Geometry: final body of the model. Coordinates: model frame, mm. A direction names the side the tool comes from. Coordinates: 2 decimals unless noted, no trailing zeros. Loops run counter-clockwise (first coordinate to the right, second up) from the corner with the lowest first, then second, coordinate; pieces in that order, holes last. Notation, with made-up numbers: (48, 7) - (70, 7) arc R13 cw to (70, 17) - close; hole circle Ø7 at (64.25, 68.5). An arc over 180 degrees is marked (long way). Put each result on its own line as item: value. Start each with the question number.
1) Section D-D on z = 30. Output: boundary loops of the cut face in (x, y).
2) Draft query along Z for faces 1 (the flat face through (5, 0, 3)), 2 (the flat face through (5, 13, 41.48)), 3 (the flat face through (-30, 16, 18.62)), 4 (the flat face through (0.86, 9, 4)). Return one class per face: +Z half, -Z half, draft (parallel to the pull), parting line (faces both ways), or undercut.
3) Section C-C on y = 17.78. Output: boundary loops of the cut face in (x, z).
4) Section A-A on y = 4.25. Output: boundary loops of the cut face in (x, z), and give its area (3 significant figures).
5) Reachability of faces 5 (the flat face through (-30, 16, 12.27)), 6 (the flat face through (5, 13, -34.72)), 7 (the flat face through (11, 9, -25.195)) from +Z, -Z, +X, -X, +Y, -Y: full face, straight path, thin tool, end or side. Return the list, or none.
6) Material intervals for line 1 along X through (y, z) = (11.5, -16); line 2 along Z through (x, y) = (-14.5, 14.25); line 3 along X through (y, z) = (12.75, 35.5), sorted ascending. Write a range as from..to.
7) Contact query for flat-ended pins moving along their axis: pin 1 Ø14 at (y, z) = (10.5, 4) entering from -X; pin 2 Ø4.5 at (y, z) = (17.78, -11.86) entering from -X; pin 3 Ø1.5 at (y, z) = (12.5, 5) entering from -X. Output: stop coordinate, or through.
8) Section B-B on x = 48.5. Output: boundary loops of the cut face in (y, z).
```python
from build123d import *

# Parameters (mm, degrees)
SKETCH1_W           = 101.6
SKETCH1_H           = 76.2
BOSS_EXTRUDE1_DEPTH = 25.4
SKETCH2_W           = 77.204847721
SKETCH2_H           = 71.12
CUT_EXTRUDE1_DEPTH  = 22.86
SKETCH3_W           = 73.394847721
SKETCH3_H           = 63.5
BOSS_EXTRUDE3_DEPTH = 12.7
SKETCH4_W           = 38.1
SKETCH4_H           = 15.24
CUT_EXTRUDE2_DEPTH  = 6.35
SKETCH7_R           = 2.535464608
CUT_EXTRUDE3_DEPTH  = 22.86
SKETCH8_W           = 6.35
SKETCH8_H           = 6.35
CUT_EXTRUDE5_DEPTH  = 17.78
SKETCH9_W           = 20.32
SKETCH9_H           = 57.15
CUT_EXTRUDE6_DEPTH  = 12.7
LPATTERN1_COUNT     = 3
LPATTERN1_PITCH     = 22.86


with BuildPart() as part:
    # Sketch1 → Boss-Extrude1 (new body)
    with BuildSketch(Plane(origin=(0, 0, 0), x_dir=(1, 0, 0), z_dir=(0, 1, 0))):
        with Locations((5.940322581, -3.37983871)):
            Rectangle(SKETCH1_W, SKETCH1_H)
    extrude(amount=BOSS_EXTRUDE1_DEPTH)

    # Sketch2 → Cut-Extrude1 (cut)
    with BuildSketch(Plane(origin=(0, 25.4, 0), x_dir=(1, 0, 0), z_dir=(0, 1, 0))):
        with Locations((15.59789872, -3.37983871)):
            Rectangle(SKETCH2_W, SKETCH2_H)
    extrude(amount=-CUT_EXTRUDE1_DEPTH, mode=Mode.SUBTRACT)

    # Sketch3 → Boss-Extrude3 (add)
    with BuildSketch(Plane(origin=(0, 2.54, 0), x_dir=(1, 0, 0), z_dir=(0, 1, 0))):
        with Locations((13.692898721, -3.37983871)):
            Rectangle(SKETCH3_W, SKETCH3_H)
    extrude(amount=BOSS_EXTRUDE3_DEPTH)

    # Sketch4 → Cut-Extrude2 (cut)
    with BuildSketch(Plane.ZY.offset(44.859677419)):
        with Locations((3.37983871, 13.97)):
            Rectangle(SKETCH4_W, SKETCH4_H)
    extrude(amount=-CUT_EXTRUDE2_DEPTH, mode=Mode.SUBTRACT)

    # Sketch7 → Cut-Extrude3 (cut)
    with BuildSketch(Plane.ZY.offset(44.859677419)):
        with Locations((-11.86016129, 17.78)):
            Circle(SKETCH7_R)
    extrude(amount=-CUT_EXTRUDE3_DEPTH, mode=Mode.SUBTRACT)

    # Sketch8 → Cut-Extrude5 (cut)
    with BuildSketch(Plane.ZY.offset(38.509677419)):
        with Locations((15.44483871, 15.875)):
            Rectangle(SKETCH8_W, SKETCH8_H)
    extrude(amount=-CUT_EXTRUDE5_DEPTH, mode=Mode.SUBTRACT)

    # Sketch9 → Cut-Extrude6 (cut)
    with BuildSketch(Plane(origin=(0, 15.24, 0), x_dir=(1, 0, 0), z_dir=(0, 1, 0))):
        with Locations((33.880322581, -3.37983871)):
            Rectangle(SKETCH9_W, SKETCH9_H)
    cut_extrude6 = extrude(amount=-CUT_EXTRUDE6_DEPTH, mode=Mode.SUBTRACT)

    # LPattern1: Cut-Extrude6 ×3
    with Locations(*[(-i * LPATTERN1_PITCH, 0, 0) for i in range(1, LPATTERN1_COUNT)]):
        add(cut_extrude6, mode=Mode.SUBTRACT)


solid = part.part
```
Answer block:
1. outline: (-44.86, 0) - (56.74, 0) - (56.74, 25.4) - (54.2, 25.4) - (54.2, 2.54) - (50.39, 2.54) - (50.39, 15.24) - (44.04, 15.24) - (44.04, 2.54) - (23.72, 2.54) - (23.72, 15.24) - (21.18, 15.24) - (21.18, 2.54) - (0.86, 2.54) - (0.86, 15.24) - (-1.68, 15.24) - (-1.68, 2.54) - (-22, 2.54) - (-22, 15.24) - (-23, 15.24) - (-23, 25.4) - (-44.86, 25.4) - close
2. face 1: draft
2. face 2: +Z half
2. face 3: undercut
2. face 4: undercut
3. outline: (-44.86, -34.72) - (56.74, -34.72) - (56.74, 41.48) - (-44.86, 41.48) - (-44.86, 22.43) - (-38.51, 22.43) - (-38.51, 18.62) - (-23, 18.62) - (-23, 38.94) - (54.2, 38.94) - (54.2, -32.18) - (-23, -32.18) - (-23, -14.4) - (-38.51, -14.4) - (-38.51, -15.67) - (-44.86, -15.67) - close; (-38.51, -9.32) - (-23, -9.32) - (-23, 12.27) - (-38.51, 12.27) - close
4. outline: (-44.86, -34.72) - (56.74, -34.72) - (56.74, 41.48) - (-44.86, 41.48) - close; hole (-23, -32.18) - (54.2, -32.18) - (54.2, 38.94) - (-23, 38.94) - (-23, 35.13) - (50.39, 35.13) - (50.39, -28.37) - (-23, -28.37) - close; hole (-22, -25.2) - (-1.68, -25.2) - (-1.68, 31.95) - (-22, 31.95) - close; hole (0.86, -25.2) - (21.18, -25.2) - (21.18, 31.95) - (0.86, 31.95) - close; hole (23.72, -25.2) - (44.04, -25.2) - (44.04, 31.95) - (23.72, 31.95) - close
4. area: 3,430 mm²
5. face 5: -X
5. face 6: -Z, +X, -X, +Y, -Y
5. face 7: +Y
6. line 1: x = -44.86..-22, -1.68..0.86, 21.18..23.72, 44.04..50.39, 54.2..56.74
6. line 2: z = -34.72..-32.18, -28.37..-25.2, 31.95..35.13, 38.94..41.48
6. line 3: x = -44.86..-23, 54.2..56.74
7. pin 1: stops at x = -44.86
7. pin 2: stops at x = 54.2
7. pin 3: stops at x = -38.51
8. outline: (0, -34.72) - (25.4, -34.72) - (25.4, -32.18) - (2.54, -32.18) - (2.54, -28.37) - (15.24, -28.37) - (15.24, 35.13) - (2.54, 35.13) - (2.54, 38.94) - (25.4, 38.94) - (25.4, 41.48) - (0, 41.48) - close
